Geometry check sheet. Reference: the model listing, model coordinates, mm. A direction names the side the tool comes from. Coordinates: 2 decimals unless noted, no trailing zeros. Write each loop counter-clockwise with the first axis right and the second up, starting at its lowest first coordinate (ties: lowest second). Pieces come first, ordered by that corner, then holes. Notation, with made-up numbers: (33.5, 65.25) -> (57.5, 65.25) arc R22 cw to (57.5, 99.25) -> close; hole circle Ø10 at (84, 64). An arc over 180 degrees is marked (long way). Use a Markdown table: item, result.
```python
from build123d import *

# Parameters (mm, degrees)
SKETCH1_R           = 9.5
SKETCH1_R_2         = 4.4
BOSS_EXTRUDE1_DEPTH = 5
CUT_EXTRUDE1_DEPTH  = 17.748134224444225
SKETCH3_R           = 9.5
SKETCH3_R_2         = 9
CUT_EXTRUDE2_DEPTH  = 4
CHAMFER1_SIZE       = 0.7
FILLET1_R           = 0.5
FILLET2_R           = 0.6


with BuildPart() as part:
    # Sketch1 → Boss-Extrude1 (new, symmetric)
    with BuildSketch(Plane.XY):
        Circle(SKETCH1_R)
        Circle(SKETCH1_R_2, mode=Mode.SUBTRACT)
    extrude(amount=BOSS_EXTRUDE1_DEPTH, both=True)

    # Sketch2 → Cut-Extrude1 (cut, through all)
    with BuildSketch(Plane.XY.offset(5)):
        with BuildLine():
            Line((0, 9.5), (-6.506462158581922, 3.612220267457224))
            Line((-6.506462158581922, 3.612220267457224), (-5.500000000000001, 2.4999999999999996))
            Line((-5.500000000000001, 2.4999999999999996), (2.000217039706271, 9.287041067749655))
            ThreePointArc((2.000217039706271, 9.287041067749655), (1.0057608702813652, 9.446610242399696), (0, 9.5))
        make_face()
    extrude(amount=-CUT_EXTRUDE1_DEPTH, mode=Mode.SUBTRACT)

    # Sketch3 → Cut-Extrude2 (cut, symmetric)
    with BuildSketch(Plane.XY):
        Circle(SKETCH3_R)
        Circle(SKETCH3_R_2, mode=Mode.SUBTRACT)
    extrude(amount=CUT_EXTRUDE2_DEPTH, both=True, mode=Mode.SUBTRACT)

    # Chamfer1
    # the kernel refuses this chamfer: 0.7 mm, written as the material it takes off along each edge
    with BuildSketch(Plane(origin=(0, 0, 4), x_dir=(0.10274511100346817, 0.9947077169525151, 0), z_dir=(0.9947077169525151, -0.10274511100346817, 0))) as chamfer1_piece_1_section:
        Polygon((9.5, CHAMFER1_SIZE), (9.5 - CHAMFER1_SIZE, 0), (9.5, 0), align=None)
    chamfer1_piece_1 = revolve(axis=Axis((0, 0, 4), (0, 0, 1)), revolution_arc=359.64, mode=Mode.PRIVATE)
    chamfer1_piece_1 = chamfer1_piece_1 - Plane(origin=(0, 0, 4.439831857806262), x_dir=(1, 0, 0), z_dir=(0, 0, -1)) * Cylinder(9, 38, mode=Mode.PRIVATE)
    add(chamfer1_piece_1, mode=Mode.SUBTRACT)
    with BuildSketch(Plane(origin=(0, 0, -4), x_dir=(0.10274511100346817, 0.9947077169525151, 0), z_dir=(0.9947077169525151, -0.10274511100346817, 0))) as chamfer1_piece_2_section:
        Polygon((9.5 - CHAMFER1_SIZE, 0), (9.5, -CHAMFER1_SIZE), (9.5, 0), align=None)
    chamfer1_piece_2 = revolve(axis=Axis((0, 0, -4), (0, 0, 1)), revolution_arc=359.64, mode=Mode.PRIVATE)
    chamfer1_piece_2 = chamfer1_piece_2 - Plane(origin=(0, 0, -4.439831857806264), x_dir=(1, 0, 0), z_dir=(0, 0, -1)) * Cylinder(9, 38, mode=Mode.PRIVATE)
    add(chamfer1_piece_2, mode=Mode.SUBTRACT)

    # Fillet1
    fillet1_edges = [part.edges().sort_by_distance(p)[0] for p in [
        (3e-17, 9.5, 4.85),
    ]]
    fillet(fillet1_edges, radius=FILLET1_R)

    # Fillet2
    fillet2_edges = [part.edges().sort_by_distance(p)[0] for p in [
        (-5.500000000000001, 2.4999999999999996, 0),
        (-6.506462158581922, 3.612220267457224, 0),
    ]]
    fillet(fillet2_edges, radius=FILLET2_R)


solid = part.part
```
Item 1: Tool access check on faces 1 (the conical face through (-0.696, -9.109, 4.335)), 2 (the flat face through (-1.577, 6.05, 0.07)), 3 (the flat face through (2, -4.1, 5)). Record the directions out of +Z, -Z, +X, -X, +Y, -Y that give a thin tool (end or side, any length) a straight path to the whole face; none if there is none.
Answer block:
| item | result |
|---|---|
| face 1 | none |
| face 2 | +Z, -Z |
| face 3 | +Z, +X, -X, +Y, -Y |
Item 2: Mould release check, pull along X, two halves, no side actions. Record for faces 4 (the conical face through (-0.697, -9.116, -4.342)), 5 (the cylindrical face through (-6.258, 3.606, -0.07)), 6 (the flat face through (2, -4.1, -5)): +X half, -X half, draft (parallel to the pull), parting line (faces both ways), or undercut.
Answer block:
| item | result |
|---|---|
| face 4 | parting line |
| face 5 | undercut |
| face 6 | draft |
Item 3: Section check A-A on y = 0. Record the boundary of the cut face in (x, z), then the cut area to 3 significant figures.
Answer block:
| item | result |
|---|---|
| outline | (-9.5, -5) -> (-4.4, -5) -> (-4.4, 5) -> (-9.5, 5) -> (-9.5, 4.7) -> (-9, 4.2) -> (-9, -4.2) -> (-9.5, -4.7) -> close; (4.4, -5) -> (9.5, -5) -> (9.5, -4.7) -> (9, -4.2) -> (9, 4.2) -> (9.5, 4.7) -> (9.5, 5) -> (4.4, 5) -> close |
| area | 93.1 mm^2 |
Item 4: Section check C-C on x = 0. Record the boundary of the cut face in (y, z), then the cut area to 3 significant figures.
Answer block:
| item | result |
|---|---|
| outline | (-9.5, -5) -> (-4.4, -5) -> (-4.4, 5) -> (-9.5, 5) -> (-9.5, 4.7) -> (-9, 4.2) -> (-9, -4.2) -> (-9.5, -4.7) -> close; (4.4, -5) -> (7.48, -5) -> (7.48, 5) -> (4.4, 5) -> close |
| area | 77.3 mm^2 |
Item 5: Section check D-D on x = -2. Count the separate pieces of the cut face and the enclosed holes in it, then the cut area to 3 significant figures.
Answer block:
| item | result |
|---|---|
| separate pieces | 3 |
| enclosed holes | 0 |
| area | 78.0 mm^2 |
Item 6: Section check B-B on z = -1.25. Record the boundary of the cut face in (x, y), then the cut area to 3 significant figures.
Answer block:
| item | result |
|---|---|
| outline | (-6.1, 3.17) arc R0.6 cw to (-6.06, 4.01) -> (-1.09, 8.52) arc R0.5 ccw to (-0.93, 8.95) arc R9 ccw (long way) to (1.54, 8.87) -> (-5.06, 2.9) arc R0.6 cw to (-5.9, 2.94) -> close; hole circle Ø8.8 at (0, 0) |
| area | 181 mm^2 |
Item 7: Depth check by flat-ended pin: P1, Ø5, axis at x = 4, z = -3.5, coming from the -Y side; P2, Ø3, axis at y = -7, z = -3.5, coming from the -X side; P3, Ø3, axis at y = -2.5, z = 3, coming from the +X side. Enter the tip coordinate at first touch or a pass-through.
Answer block:
| item | result |
|---|---|
| P1 | stops at y = -9.33 |
| P2 | stops at x = -7.28 |
| P3 | stops at x = 9.01 |
Item 8: Thickness scan on L1, parallel to Y at x = -3.25, z = 3.75; L2, parallel to Y at x = 3, z = 1.25; L3, parallel to Y at x = 0, z = -0.5. Record the ranges inside material, lowest first. Write a range as [from, to].
Answer block:
| item | result |
|---|---|
| L1 | y = [-8.39, -2.97], [2.97, 4.54], [6.56, 8.39] |
| L2 | y = [-8.49, -3.22], [3.22, 8.49] |
| L3 | y = [-9, -4.4], [4.4, 7.48] |
